Read the model definition and answer for the solid it produces. Units are mm, in the model's axes. A direction names the side the tool comes from. Round coordinates to 2 decimals unless told otherwise and drop trailing zeros. Write each loop counter-clockwise with the first axis right and the second up, starting at its lowest first coordinate (ties: lowest second). Pieces come first, ordered by that corner, then holes. Notation, with made-up numbers: (-18.5, 49) -> (23.5, 49) arc R4 cw to (23.5, 55) -> close; hole circle Ø4 at (87.25, -14.5). An arc over 180 degrees is marked (long way). Return JSON: item names as keys, results as strings. Group by question number.
(1) The mould has two halves that part along X. Classify faces 1 (the flat face through (-136, 49, 0)), 2 (the cylindrical face through (-198.2, 39.61, 0.68)), 3 (the cylindrical face through (-73.63, 27.68, 249.32)): released by +X, released by -X, zero draft, split by the parting line, or undercut.
(2) Given pin 1 (2 mm diameter, centred on x = -50, y = 1, fed in from -Z); pin 2 (1.5 mm diameter, centred on y = 45, z = 165.5, fed in from +X); pin 3 (0.6 mm diameter, centred on y = 1, z = 153, fed in from -X); pin 4 (3 mm diameter, centred on x = -121.5, y = 28, fed in from -Z), each flat-ended and moving along its own axis, determine where each tip first touches the part or whether it passes through.
(3) A cutting plane is placed at A-A on z = 129.5. Give the vertices of the cut face in (x, y), then the cut area to 4 significant figures.
(4) For faces 4 (the flat face through (-91, 0, 151)), 5 (the flat face through (-55.955, 45.991, 123.278)), 6 (the cylindrical face through (-73.697, 27.428, 0.68)), determine the directions among +Z, -Z, +X, -X, +Y, -Y from which every point of the face is accessible in a straight line to the end or side of a thin tool.
(5) A cutting plane is placed at B-B on y = 28.5. State how many separate pieces and enclosed holes the cut face has, then the cut area to 3 significant figures.
(6) Straight lines are drawn through the part: line 1 (Z direction, x = -211, y = 42.5); line 2 (X direction, y = 1.5, z = 96.25); line 3 (X direction, y = 0.8, z = 153.75). For each, find the intervals that lie inside material, in ascending order.
```python
from build123d import *

# Parameters (mm, degrees)
EXTRUDE_1_DEPTH           = 250
SHELL_1_T                 = -2
SKETCH_4_R                = 40
CUT_EXTRUDE_3_DEPTH       = 42
SKETCH_6_R                = 40
CUT_EXTRUDE_5_DEPTH       = 42
SKETCH_7_R                = 1.5
SKETCH_7_W                = 3.5
SKETCH_7_H                = 20
SKETCH_7_W_2              = 12
SKETCH_7_W_3              = 20
SKETCH_7_H_2              = 12
CUT_EXTRUDE_6_DEPTH       = 32
SKETCH_8_W                = 50
SKETCH_8_H                = 50
CUT_EXTRUDE_7_DEPTH       = 15
SKETCH_9_W                = 50
SKETCH_9_H                = 48
CUT_EXTRUDE_8_DEPTH       = 15
SKETCH_10_W               = 70
SKETCH_10_H               = 25
CUT_EXTRUDE_9_DEPTH       = 2
SKETCH_13_W               = 25
SKETCH_13_H               = 49.428785774
CUT_EXTRUDE_10_DEPTH      = 304
SKETCH_14_W               = 66.85616243
SKETCH_14_H               = 25
CUT_EXTRUDE_11_DEPTH      = 2
SKETCH_15_W               = 3
SKETCH_15_H               = 20
SKETCH_15_W_2             = 20
SKETCH_15_H_2             = 3
CUT_EXTRUDE_12_DEPTH      = 2
SKETCH_16_R               = 1.5
CUT_EXTRUDE_13_DEPTH      = 90
SKETCH_18_R               = 1.6
CUT_EXTRUDE_14_DEPTH      = 5
CUT_EXTRUDE_15_DEPTH      = 264
SKETCH_20_W               = 250
SKETCH_20_H               = 17.277243338
EXTRUDE_2_DEPTH           = 2
SKETCH_21_R               = 1.5
CUT_EXTRUDE_17_DEPTH      = 1
CUT_EXTRUDE_17_DEPTH_BACK = 251


with BuildPart() as part:
    # 草图1 → 凸台-拉伸1 (new body)
    with BuildSketch(Plane.XY):
        Polygon((0, 0), (-185, 0), (-256.697410121, 62.325607754), (-71.697410121, 62.325607754), align=None)
    extrude(amount=EXTRUDE_1_DEPTH)

    # 抽壳1
    shell_1_openings = [part.faces().sort_by_distance(p)[0] for p in [
        (-164.197410121, 62.325607754, 125),
    ]]
    offset(amount=SHELL_1_T, openings=shell_1_openings, kind=Kind.INTERSECTION)

    # 草图4 → 切除-拉伸3 (cut)
    with BuildSketch(Plane.XY.offset(250)):
        with Locations((-35, 17.3)):
            Circle(SKETCH_4_R)
        with Locations((-165, 17.3)):
            Circle(SKETCH_4_R)
    extrude(amount=-CUT_EXTRUDE_3_DEPTH, mode=Mode.SUBTRACT)

    # 草图6 → 切除-拉伸5 (cut)
    with BuildSketch(Plane(origin=(0, 0, 0), x_dir=(-1, 0, 0), z_dir=(0, 0, -1))):
        with Locations((165, 17.3)):
            Circle(SKETCH_6_R)
        with BuildLine():
            ThreePointArc((15.18510716, -17.447230418), (75, 17.3), (15.18510716, 52.047230418))
            ThreePointArc((15.18510716, 52.047230418), (-45.184680822, 17.3), (15.18510716, -17.447230418))
        make_face()
    extrude(amount=-CUT_EXTRUDE_5_DEPTH, mode=Mode.SUBTRACT)

    # 草图7 → 切除-拉伸6 (cut)
    with BuildSketch(Plane(origin=(0, 2, 0), x_dir=(1, 0, 0), z_dir=(0, 1, 0))):
        with Locations((-95.174280419, -111.75)):
            Circle(SKETCH_7_R)
        with Locations((-95.174280419, -138.25)):
            Circle(SKETCH_7_R)
        with Locations((-11.41, -96.25)):
            Circle(SKETCH_7_R)
        with Locations((-37.91, -96.25)):
            Circle(SKETCH_7_R)
        with Locations((-37.91, -153.75)):
            Circle(SKETCH_7_R)
        with Locations((-11.41, -153.75)):
            Circle(SKETCH_7_R)
        with Locations((-174.09, -196.75)):
            Rectangle(SKETCH_7_W, SKETCH_7_H)
        with Locations((-25.41, -196.75)):
            Rectangle(SKETCH_7_W, SKETCH_7_H)
        with Locations((-163.59, -196.75)):
            Rectangle(SKETCH_7_W, SKETCH_7_H)
        with Locations((-134.59, -196.75)):
            Rectangle(SKETCH_7_W, SKETCH_7_H)
        with Locations((-35.91, -196.75)):
            Rectangle(SKETCH_7_W, SKETCH_7_H)
        with Locations((-64.91, -196.75)):
            Rectangle(SKETCH_7_W, SKETCH_7_H)
        with Locations((-134.59, -53.25)):
            Rectangle(SKETCH_7_W, SKETCH_7_H)
        with Locations((-163.59, -53.25)):
            Rectangle(SKETCH_7_W, SKETCH_7_H)
        with Locations((-174.09, -53.25)):
            Rectangle(SKETCH_7_W, SKETCH_7_H)
        with Locations((-64.91, -53.25)):
            Rectangle(SKETCH_7_W, SKETCH_7_H)
        with Locations((-35.91, -53.25)):
            Rectangle(SKETCH_7_W, SKETCH_7_H)
        with Locations((-25.41, -53.25)):
            Rectangle(SKETCH_7_W, SKETCH_7_H)
        with Locations((-95.174280419, -125)):
            Rectangle(SKETCH_7_W_2, SKETCH_7_H)
        with Locations((-24.66, -96.25)):
            Rectangle(SKETCH_7_W_3, SKETCH_7_H_2)
        with Locations((-24.66, -153.75)):
            Rectangle(SKETCH_7_W_3, SKETCH_7_H_2)
    extrude(amount=-CUT_EXTRUDE_6_DEPTH, mode=Mode.SUBTRACT)

    # 草图8 → 切除-拉伸7 (cut)
    with BuildSketch(Plane.XY.offset(208)):
        with Locations((-25, 27)):
            Rectangle(SKETCH_8_W, SKETCH_8_H)
    extrude(amount=-CUT_EXTRUDE_7_DEPTH, mode=Mode.SUBTRACT)

    # 草图9 → 切除-拉伸8 (cut)
    with BuildSketch(Plane(origin=(0, 0, 42), x_dir=(-1, 0, 0), z_dir=(0, 0, -1))):
        with Locations((25, 26)):
            Rectangle(SKETCH_9_W, SKETCH_9_H)
    extrude(amount=-CUT_EXTRUDE_8_DEPTH, mode=Mode.SUBTRACT)

    # 草图10 → 切除-拉伸9 (cut)
    with BuildSketch(Plane(origin=(0, 0, 0), x_dir=(0.75470958, -0.656059029, 0), z_dir=(0.656059029, 0.75470958, 0))):
        with Locations((-35, -182.5)):
            Rectangle(SKETCH_10_W, SKETCH_10_H)
        with Locations((-35, -67.5)):
            Rectangle(SKETCH_10_W, SKETCH_10_H)
        with Locations((-35, -125)):
            Rectangle(SKETCH_10_W, SKETCH_10_H)
    extrude(amount=-CUT_EXTRUDE_9_DEPTH, mode=Mode.SUBTRACT)

    # 草图13 → 切除-拉伸10 (cut)
    with BuildSketch(Plane(origin=(0, 0, 0), x_dir=(-1, 0, 0), z_dir=(0, 0, -1))):
        with Locations((101.10376969, 26.714392887)):
            Rectangle(SKETCH_13_W, SKETCH_13_H)
    extrude(amount=-CUT_EXTRUDE_10_DEPTH, mode=Mode.SUBTRACT)

    # 草图14 → 切除-拉伸11 (cut)
    with BuildSketch(Plane(origin=(-78.314370103, -90.090377198, 0), x_dir=(0.75470958, -0.656059029, 0), z_dir=(0.656059029, 0.75470958, 0))):
        with Locations((-173.797122915, -67.5)):
            Rectangle(SKETCH_14_W, SKETCH_14_H)
        with Locations((-173.797122915, -125)):
            Rectangle(SKETCH_14_W, SKETCH_14_H)
        with Locations((-173.797122915, -182.5)):
            Rectangle(SKETCH_14_W, SKETCH_14_H)
    extrude(amount=-CUT_EXTRUDE_11_DEPTH, mode=Mode.SUBTRACT)

    # 草图15 → 切除-拉伸12 (cut)
    with BuildSketch(Plane.XZ):
        with Locations((-100.462980788, 237.5)):
            Rectangle(SKETCH_15_W, SKETCH_15_H)
        with Locations((-15.456937779, 182.5)):
            Rectangle(SKETCH_15_W_2, SKETCH_15_H_2)
        with Locations((-15.548506173, 125)):
            Rectangle(SKETCH_15_W_2, SKETCH_15_H_2)
        with Locations((-15.548506173, 67.407755874)):
            Rectangle(SKETCH_15_W_2, SKETCH_15_H_2)
        with Locations((-100.787471441, 12.5)):
            Rectangle(SKETCH_15_W, SKETCH_15_H)
        with Locations((-173.064348699, 68.747523441)):
            Rectangle(SKETCH_15_W_2, SKETCH_15_H_2)
        with Locations((-173.064348699, 125)):
            Rectangle(SKETCH_15_W_2, SKETCH_15_H_2)
        with Locations((-173.064348699, 182.5)):
            Rectangle(SKETCH_15_W_2, SKETCH_15_H_2)
    extrude(amount=-CUT_EXTRUDE_12_DEPTH, mode=Mode.SUBTRACT)

    # 草图16 → 切除-拉伸13 (cut)
    with BuildSketch(Plane(origin=(-1.312118058, -1.50941916, 0), x_dir=(0.75470958, -0.656059029, 0), z_dir=(-0.656059029, -0.75470958, 0))):
        with Locations((-22.161189798, 96.25)):
            Circle(SKETCH_16_R)
        with Locations((-36.461189798, 96.25)):
            Circle(SKETCH_16_R)
        with Locations((-22.161189798, 153.75)):
            Circle(SKETCH_16_R)
        with Locations((-36.461189798, 153.75)):
            Circle(SKETCH_16_R)
    extrude(amount=-CUT_EXTRUDE_13_DEPTH, mode=Mode.SUBTRACT)

    # 草图18 → 切除-拉伸14 (cut)
    with BuildSketch(Plane(origin=(0, 0, 0), x_dir=(0.75470958, -0.656059029, 0), z_dir=(0.656059029, 0.75470958, 0))):
        with Locations((-69.177168292, -200.735802704)):
            Circle(SKETCH_18_R)
        with Locations((-69.177168292, -49.264197296)):
            Circle(SKETCH_18_R)
    extrude(amount=-CUT_EXTRUDE_14_DEPTH, mode=Mode.SUBTRACT)

    # 草图19 → 切除-拉伸15 (cut)
    with BuildSketch(Plane.XY.offset(250)):
        Polygon((-256.697410121, 62.325607754), (-241.697410121, 62.325607754), (-230.362518633, 62.325607754), (-241.697410121, 49.286306687), align=None)
    extrude(amount=-CUT_EXTRUDE_15_DEPTH, mode=Mode.SUBTRACT)

    # 草图20 → 凸台-拉伸2 (add)
    with BuildSketch(Plane(origin=(-162.07092196, 140.886103045, 0), x_dir=(0, 0, 1), z_dir=(-0.75470958, 0.656059029, 0))):
        with Locations((125, -112.732298694)):
            Rectangle(SKETCH_20_W, SKETCH_20_H)
    extrude(amount=EXTRUDE_2_DEPTH)

    # 草图21 → 切除-拉伸17 (cut, two sides)
    with BuildSketch(Plane.XY.offset(250)) as cut_extrude_17_sk:
        with Locations((-78.60376969, 54.325607754)):
            Circle(SKETCH_21_R)
        with Locations((-220.362518633, 54.325607754)):
            Circle(SKETCH_21_R)
    extrude(amount=CUT_EXTRUDE_17_DEPTH, mode=Mode.SUBTRACT)
    extrude(cut_extrude_17_sk.sketch, amount=-CUT_EXTRUDE_17_DEPTH_BACK, mode=Mode.SUBTRACT)


solid = part.part
```
Checks:
{
 "1": {"face 1": "zero draft", "face 2": "undercut", "face 3": "released by +X"},
 "2": {"pin 1": "stops at z = 42", "pin 2": "stops at x = -50.9", "pin 3": "stops at x = -186.5", "pin 4": "stops at z = 0"},
 "3": {"outline": "(-243.21, 50.6) -> (-236.02, 44.35) -> (-234.71, 45.86) -> (-240.39, 50.8) -> (-230.36, 62.33) -> (-231.87, 63.64) -> close; (-185.56, 0.49) -> (-185, 0) -> (-101.17, 0) -> (-101.17, 2) -> (-184.25, 2) -> close; (-89.17, 0) -> (-3.05, 0) -> (-5.35, 2) -> (-89.17, 2) -> close; (-74.75, 62.33) -> (-54.14, 44.41) -> (-52.83, 45.92) -> (-71.7, 62.33) -> close", "area": "439.5 mm^2"},
 "4": {"face 4": "+Z, -Z, +X, -X, -Y", "face 5": "none", "face 6": "-Z, +X"},
 "5": {"separate pieces": "10", "enclosed holes": "0", "area": "890 mm^2"},
 "6": {"line 1": "z = 0 to 2, 248 to 250", "line 2": "x = -186.73 to -39.41, -36.41 to -34.66, -14.66 to -12.91, -9.91 to -1.73", "line 3": "x = -185.92 to -39.41, -36.41 to -34.66, -14.66 to -12.91, -9.91 to -0.92"}
}
